Check sheet for the modelled part. Datum: model origin and axes. Units: mm. A direction names the side the tool comes from. Give positions to 0.01 mm unless a question says otherwise; leave off trailing zeros. Write each loop counter-clockwise with the first axis right and the second up, starting at its lowest first coordinate (ties: lowest second). Pieces come first, ordered by that corner, then holes. Notation, with made-up numbers: (85.5, 22.5) -> (128.5, 22.5) arc R30 cw to (128.5, 44.5) -> close; hole circle Ø8 at (70, 79). An arc over 180 degrees is marked (long way). Use a Markdown table: item, result. Add a question column.
1. Cross-section at D-D (y = 5.75). Enter the section's corners in (x, z), then the cut area to 3 significant figures.
2. Scan lines: probe 1 along X at (y, z) = (18.25, 0); probe 2 along Y at (x, z) = (-13, -10.5); probe 3 along X at (y, z) = (10.75, 0). Record each from-to range of solid material in increasing order. Write a range as [from, to].
3. Set-up check for faces 1 (the cylindrical face through (-10.648, 0.743, -13.887)), 2 (the cylindrical face through (9.7, 19.06, 6.18)), 3 (the flat face through (-11.42, 1.5, 11.42)): record each of +Z, -Z, +X, -X, +Y, -Y from which the full face is reachable in a straight line by a thin tool's end or side.
4. Gauge pin test, flat ends, axial feed: P1, Ø5, axis at y = 8, z = -11.5, coming from the +X side; P2, Ø4, axis at x = -12, y = 16.5, coming from the -Z side; P3, Ø3, axis at y = 22.5, z = -12, coming from the -X side. Record the tip position at first contact, or that the pin passes through.
5. Cross-section at C-C (y = 23.25). Enter the section's corners in (x, z), then the cut area to 3 significant figures.
6. Release check for a two-part mould opening along Y. For faces 4 (the flat face through (-4, 0, 4)), 5 (the flat face through (0, 25, 5)), 6 (the cylindrical face through (-15.62, 6.92, -3.47)), 7 (the flat face through (-11.42, 12.5, 11.42)) record: released by +Y, released by -Y, zero draft, split by the parting line, or undercut.
from build123d import *

# Parameters (mm, degrees)
SKETCH1_R               = 17.5
BOSS_EXTRUDE1_DEPTH     = 1.5
SKETCH2_R               = 16
BOSS_EXTRUDE2_DEPTH     = 11
SKETCH3_R               = 17.5
BOSS_EXTRUDE3_DEPTH     = 1.5
SKETCH4_R               = 11.5
BOSS_EXTRUDE4_DEPTH     = 11
CUT_EXTRUDE1_DEPTH      = 36.178118199
CUT_EXTRUDE1_DEPTH_BACK = 36.178118199
SKETCH6_R               = 4
CHAMFER1_SIZE           = 1
CHAMFER2_SIZE           = 0.25
FILLET1_R               = 0.25


with BuildPart() as part:
    # Sketch1 → Boss-Extrude1 (new body)
    with BuildSketch(Plane(origin=(0, 0, 0), x_dir=(1, 0, 0), z_dir=(0, 1, 0))):
        with Locations(Location((0, 0, 0), (0, 0, 270))):
            Circle(SKETCH1_R)
    extrude(amount=BOSS_EXTRUDE1_DEPTH)

    # Sketch2 → Boss-Extrude2 (add)
    with BuildSketch(Plane(origin=(0, 1.5, 0), x_dir=(1, 0, 0), z_dir=(0, 1, 0))):
        with Locations(Location((0, 0, 0), (0, 0, 270))):
            Circle(SKETCH2_R)
    extrude(amount=BOSS_EXTRUDE2_DEPTH)

    # Sketch3 → Boss-Extrude3 (add)
    with BuildSketch(Plane(origin=(0, 12.5, 0), x_dir=(1, 0, 0), z_dir=(0, 1, 0))):
        with Locations(Location((0, 0, 0), (0, 0, 270))):
            Circle(SKETCH3_R)
    extrude(amount=BOSS_EXTRUDE3_DEPTH)

    # Sketch4 → Boss-Extrude4 (add)
    with BuildSketch(Plane(origin=(0, 14, 0), x_dir=(1, 0, 0), z_dir=(0, 1, 0))):
        with Locations(Location((0, 0, 0), (0, 0, 270))):
            Circle(SKETCH4_R)
    extrude(amount=BOSS_EXTRUDE4_DEPTH)

    # Sketch6 → Cut-Extrude1 (cut, two sides: drawn at the far end of the back side and taken through both)
    with BuildSketch(Plane(origin=(0, 25, 0), x_dir=(1, 0, 0), z_dir=(0, 1, 0)).offset(-CUT_EXTRUDE1_DEPTH_BACK)):
        with Locations(Location((0, 0, 0), (0, 0, 270))):
            Circle(SKETCH6_R)
    extrude(amount=CUT_EXTRUDE1_DEPTH + CUT_EXTRUDE1_DEPTH_BACK, mode=Mode.SUBTRACT)

    # Chamfer1
    chamfer1_edges = [part.edges().sort_by_distance(p)[0] for p in [
        (0, 25, -11.5),
    ]]
    chamfer(chamfer1_edges, length=CHAMFER1_SIZE)

    # Chamfer2
    chamfer2_edges = [part.edges().sort_by_distance(p)[0] for p in [
        (0, 0, -17.5),
        (0, 1.5, -17.5),
        (0, 12.5, -17.5),
        (0, 14, -17.5),
    ]]
    chamfer(chamfer2_edges, length=CHAMFER2_SIZE)

    # Fillet1
    fillet1_edges = [part.edges().sort_by_distance(p)[0] for p in [
        (0, 14, -11.5),
    ]]
    fillet(fillet1_edges, radius=FILLET1_R)


solid = part.part
Worked answers:
| question | item | result |
|---|---|---|
| 1 | outline | circle Ø32 at (0, 0); hole circle Ø8 at (0, 0) |
| 1 | area | 754 mm² |
| 2 | probe 1 | x = [-11.5, -4], [4, 11.5] |
| 2 | probe 2 | y = [0, 1.5], [12.5, 14] |
| 2 | probe 3 | x = [-16, -4], [4, 16] |
| 3 | face 1 | +Y, -Y |
| 3 | face 2 | +Y |
| 3 | face 3 | none |
| 4 | P1 | stops at x = 13.23 |
| 4 | P2 | stops at z = -5.68 |
| 4 | P3 | stops at x = -4.69 |
| 5 | outline | circle Ø23 at (0, 0); hole circle Ø8 at (0, 0) |
| 5 | area | 365 mm² |
| 6 | face 4 | released by -Y |
| 6 | face 5 | released by +Y |
| 6 | face 6 | undercut |
| 6 | face 7 | undercut |
